Autodesk Inventor part; units mm, degrees
ref_plane "YZ Plane" through (0, 0, 0) normal (1, 0, 0) x (0, 1, 0)
ref_plane "XZ Plane" through (0, 0, 0) normal (0, 1, 0) x (-1, 0, 0)
ref_plane "XY Plane" through (0, 0, 0) normal (0, 0, 1) x (1, 0, 0)
sketch "Szkic1" plane through (0, 0, 0) normal (0, 1, 0) x (-1, 0, 0)
  line L0 (-2.85, 7.85) -> (2.85, 7.85)
  line L1 (2.85, 7.85) -> (2.85, -7.85)
  line L2 (2.85, -7.85) -> (-2.85, -7.85)
  line L3 (-2.85, -7.85) -> (-2.85, 7.85)
  line L4 (-2.85, 7.85) -> (2.85, -7.85) construction
  line L5 (2.85, 7.85) -> (-2.85, -7.85) construction
  line L6 (-2.85, 2) -> (-4.55, 2)
  line L7 (-4.55, 2) -> (-4.55, -2)
  line L8 (-4.55, -2) -> (-2.85, -2)
  line L9 (-2.85, -2) -> (-2.85, 2)
  point P0 (0, 0)
  dimension "d0" = 15.7
  dimension "d1" = 5.7
  dimension "d2" = 4
  dimension "d3" = 7.4
  dimension "d4" = 2
extrude "Wyciągnięcie proste1" add sketch "Szkic1" along normal blind 10.5
sketch "Szkic2" plane through (0, 10.5, 0) normal (0, 1, 0) x (1, 0, 0)
  line L0 (-3.45, -9.1) -> (4.05, -9.1)
  line L1 (4.05, -9.1) -> (4.05, 9.1)
  line L2 (4.05, 9.1) -> (-3.45, 9.1)
  line L3 (-3.45, 9.1) -> (-3.45, -9.1)
  line L4 (-3.45, -9.1) -> (4.05, 9.1) construction
  line L5 (4.05, -9.1) -> (-3.45, 9.1) construction
  line L6 (-2.85, 7.85) -> (-2.85, -7.85)
  line L7 (2.85, 2) -> (2.85, 7.85)
  point P0 (0, 0)
  point P1 (0.3, 0)
  point P2 (0.3, 0)
  dimension "d7" = 18.2
  dimension "d8" = 7.5
  dimension "d10" = 1.2
extrude "Wyciągnięcie proste2" add sketch "Szkic2" along normal blind 8
properties part number "Connector_female" material "Tworzywo sztuczne ABS"
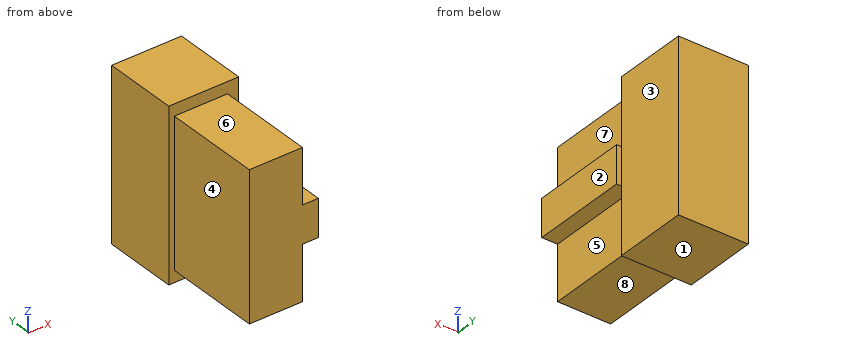
Could you check a few things on this model? Use its own coordinates, in mm. Face numbers are marked on the shaded views. A direction names the side the tool comes from. Give positions to 0.01 mm unless a question says otherwise; leave off trailing zeros. Write each loop counter-clockwise with the first axis right and the second up, starting at its lowest first coordinate (ties: lowest second). Pieces come first, ordered by that corner, then holes. Notation, with made-up numbers: (80, 82.25) -> (128, 82.25) arc R19 ccw to (128, 89.25) -> close; hole circle Ø10 at (-19.5, 57). An arc over 180 degrees is marked (long way). Write each question's results on one line, items separated by ' | '. Start each with the question number.
Q1. Suppose I cut it at A-A, the plane x = 2.5. List the corners of the cut face in (y, z) for me.
Q2. Which directions (+Z, -Z, +X, -X, +Y, -Y) give clear straight access to the entire face, cutting with the end or side of a thin tool? Please do the marked faces 1, 2, 3, 4 and 5.
Q3. Suppose I cut it at C-C, the plane y = 11.5. List the corners of the cut face in (x, z) for me.
Q4. Suppose I cut it at B-B, the plane z = 1. List the corners of the cut face in (x, y) for me.
Q5. We'd pull the mould along Z, two halves only. Please class the marked faces 6, 7 and 8: +Z half, -Z half, draft (parallel to the pull), parting line (faces both ways), or undercut.
Q6. I'm going to push flat-ended pins straight in: pin 1 Ø0.5 at (x, y) = (3.5, 6.5) entering from +Z; pin 2 Ø1.5 at (x, y) = (-1, 9) entering from -Z; pin 3 Ø6 at (y, z) = (9, -5.5) entering from -X; pin 4 Ø6 at (y, z) = (15, -6) entering from +X. Where does each tip first touch, or does it pass through?
Q7. I need wall thicknesses on probe 1 along X at (y, z) = (15.75, 3.25); probe 2 along Z at (x, y) = (0, 3.75); probe 3 along X at (y, z) = (9.75, 4.25). Which ranges of each line are inside material? Lowest first, please.
Outcome:
1) outline: (0, -7.85) -> (10.5, -7.85) -> (10.5, -9.1) -> (18.5, -9.1) -> (18.5, 9.1) -> (10.5, 9.1) -> (10.5, 7.85) -> (0, 7.85) -> close
2) face 1: -Z, +X, -X, +Y, -Y | face 2: +Z, -Z, +X, +Y, -Y | face 3: +Z, -Z, +X, +Y | face 4: +Z, -Z, -X, -Y | face 5: -Z, +X, -Y
3) outline: (-3.45, -9.1) -> (4.05, -9.1) -> (4.05, 9.1) -> (-3.45, 9.1) -> close
4) outline: (-3.45, 10.5) -> (-2.85, 10.5) -> (-2.85, 0) -> (4.55, 0) -> (4.55, 10.5) -> (4.05, 10.5) -> (4.05, 18.5) -> (-3.45, 18.5) -> close
5) face 6: +Z half | face 7: draft | face 8: -Z half
6) pin 1: z = 2 | pin 2: z = -7.85 | pin 3: x = -3.45 | pin 4: x = 4.05
7) probe 1: -3.45 to 4.05 | probe 2: -7.85 to 7.85 | probe 3: -2.85 to 2.85
